The listing builds one solid part. Answer for the finished solid, in the listing's coordinates (mm). A direction names the side the tool comes from. Round coordinates to 2 decimals unless told otherwise and drop trailing zeros. Write each loop counter-clockwise with the first axis right and the second up, starting at its lowest first coordinate (ties: lowest second). Pieces come first, ordered by that corner, then holes. Notation, with made-up numbers: (76.25, 72.25) - (134.25, 72.25) arc R17 cw to (134.25, 97.25) - close; hole circle Ø2 at (-32, 66). An arc over 180 degrees is marked (long way). Return JSON: item names as keys, results as strings. Group by question number.
(1) Section A-A, the plane y = -0.5 is taken. Write down the section's boundary in (x, z).
(2) Which of the six approach directions +Z, -Z, +X, -X, +Y, -Y give full straight-line access (tool end or side, diameter ignored) to faces 4 (the flat face through (-3, 27, -1.4)), 5 (the flat face through (1.4, -2, 3)), 6 (the flat face through (-1.4, 27, -3)), 7 (the flat face through (0, 12, -2))?
(3) Section C-C, the plane z = -2 is taken. Write down the section's boundary in (x, y).
(4) Section D-D, the plane y = 3.5 is taken. Write down the section's boundary in (x, z).
(5) Find the intervals of material crossed by line 1 along X through (y, z) = (27, 2); line 2 along Z through (x, y) = (2.5, 1.5); line 3 along Y through (x, z) = (-1, 1.75), in increasing order. Write a range as [from, to].
(6) Section B-B, the plane x = 4 is taken. Write down the section's boundary in (y, z), then the cut area to 3 significant figures.
(7) Each of these flat-tipped pins is pushed along its axis until it touches: pin 1 (1.8 mm diameter, centred on x = 4, y = 26.5, fed in from -Z); pin 2 (1.8 mm diameter, centred on y = 27, z = -3.5, fed in from +X); pin 3 (1.1 mm diameter, centred on x = -3.5, y = 27.5, fed in from +Z); pin 4 (4 mm diameter, centred on x = 4, z = -2.5, fed in from -Y). Where does it stop, or does it pass through?
(8) Determine the mould class of faces 1 (the flat face through (3, -2, 1.4)), 2 (the flat face through (-3, -2, -1.4)), 3 (the flat face through (-1, 0, 1)) for opening direction Z: +Z half, -Z half, draft (parallel to the pull), parting line (faces both ways), or undercut.
```python
from build123d import *

# Parameters (mm, degrees)
BOSS_EXTRUDE2_DEPTH = 25
SKETCH13_W          = 3.6
SKETCH13_H          = 3.6
BOSS_EXTRUDE3_DEPTH = 4
SKETCH15_W          = 3.6
SKETCH15_H          = 3.6
BOSS_EXTRUDE4_DEPTH = 4


with BuildPart() as part:
    # Sketch12 → Boss-Extrude2 (new body)
    with BuildSketch(Plane(origin=(0, 0, 0), x_dir=(1, 0, 0), z_dir=(0, 1, 0))):
        Polygon((-5, -5), (5, -5), (5, 0), (0, 0), (0, 5), (-5, 5), (-5, 0), align=None)
    extrude(amount=BOSS_EXTRUDE2_DEPTH)

    # Sketch13 → Boss-Extrude3 (add)
    with BuildSketch(Plane(origin=(0, 0, 0), x_dir=(1, 0, 0), z_dir=(0, 1, 0))):
        with Locations((-3.2, 3.2)):
            Rectangle(SKETCH13_W, SKETCH13_H)
        with Locations((3.2, -3.2)):
            Rectangle(SKETCH13_W, SKETCH13_H)
    extrude(amount=-BOSS_EXTRUDE3_DEPTH)

    # Sketch15 → Boss-Extrude4 (add)
    with BuildSketch(Plane(origin=(0, 25, 0), x_dir=(1, 0, 0), z_dir=(0, 1, 0))):
        with Locations((-3.2, 3.2)):
            Rectangle(SKETCH15_W, SKETCH15_H)
        with Locations((3.2, -3.2)):
            Rectangle(SKETCH15_W, SKETCH15_H)
    extrude(amount=BOSS_EXTRUDE4_DEPTH)


solid = part.part
```
Working result:
{
 "1": {"outline": "(-5, -5) - (-1.4, -5) - (-1.4, -1.4) - (-5, -1.4) - close; (1.4, 1.4) - (5, 1.4) - (5, 5) - (1.4, 5) - close"},
 "2": {"face 4": "+Z, +X, -X, +Y", "face 5": "+Z, -Z, -X, -Y", "face 6": "+Z, -Z, +X, +Y", "face 7": "-Z, +X, +Y, -Y"},
 "3": {"outline": "(-5, -4) - (-1.4, -4) - (-1.4, 0) - (0, 0) - (0, 25) - (-1.4, 25) - (-1.4, 29) - (-5, 29) - close"},
 "4": {"outline": "(-5, -5) - (0, -5) - (0, 0) - (5, 0) - (5, 5) - (-5, 5) - close"},
 "5": {"line 1": "x = [1.4, 5]", "line 2": "z = [0, 5]", "line 3": "y = [0, 25]"},
 "6": {"outline": "(-4, 1.4) - (0, 1.4) - (0, 0) - (25, 0) - (25, 1.4) - (29, 1.4) - (29, 5) - (-4, 5) - close", "area": "154 mm^2"},
 "7": {"pin 1": "stops at z = 1.4", "pin 2": "stops at x = -1.4", "pin 3": "stops at z = -1.4", "pin 4": "passes through"},
 "8": {"face 1": "-Z half", "face 2": "+Z half", "face 3": "draft"}
}
